Autodesk Inventor part; units mm, degrees
ref_plane "Work Plane1" through (0, -12, 0) normal (0, 1, 0) x (1, 0, 0)
ref_plane "YZ Plane" through (0, 0, 0) normal (1, 0, 0) x (0, 1, 0)
ref_plane "XZ Plane" through (0, 0, 0) normal (0, 1, 0) x (-1, 0, 0)
sketch "Sketch1" plane through (0, 0, 0) normal (0, 1, 0) x (-1, 0, 0)
  line L0 (0, 0) -> (35, 0)
  line L1 (35, 0) -> (35, 40)
  line L2 (35, 40) -> (0, 40)
  line L3 (0, 40) -> (0, 0)
  line L4 (50, 0) -> (85, 0)
  line L5 (85, 0) -> (85, 40)
  line L6 (85, 40) -> (50, 40)
  line L7 (50, 40) -> (50, 0)
  line L8 (50, 40) -> (35, 40)
  line L9 (50, 0) -> (35, 0)
  line L10 (0, 40) -> (0, 51)
  line L11 (0, 51) -> (85, 51)
  line L12 (85, 51) -> (85, 40)
  dimension "d0" = 40
  dimension "d1" = 35
  dimension "d2" = 40
  dimension "d3" = 35
  dimension "d4" = 50
  dimension "d5" = 0
  dimension "d6" = 11
extrude "Extrusion1" add sketch "Sketch1" along normal blind 30
sketch "Sketch2" plane through (0, 0, 0) normal (0, -1, 0) x (1, 0, 0)
  line L0 (-85, 0) -> (-85, 51)
  line L1 (0, 0) -> (-85, 0)
  line L2 (0, 51) -> (0, 0)
  line L3 (-85, 51) -> (0, 51)
  line L4 (-85, 51) -> (0, 51)
  line L5 (-85, 0) -> (-85, 51)
  line L6 (0, 51) -> (-85, 51)
  line L7 (-85, 51) -> (-85, 41)
  line L8 (-85, 41) -> (0, 41)
  line L9 (0, 41) -> (0, 51)
  dimension "d9" = 10
extrude "Extrusion2" add sketch "Sketch2" along normal blind 12 contours L0 L3 L2 L8
sketch "Sketch3" plane through (0, 0, 0) normal (0, 0, -1) x (-1, 0, 0)
  line L0 (0, 0) -> (85, 0)
  line L1 (85, 0) -> (85, 30)
  line L2 (0, 30) -> (85, 30)
  line L3 (0, 0) -> (0, 30)
  circle A0 centre (17.5, 10) radius 5.25
  circle A1 centre (67.5, 10) radius 5.25
  dimension "d12" = 10.5
  dimension "d13" = 10.5
  dimension "d14" = 10
  dimension "d15" = 10
  dimension "d16" = 50
  dimension "d17" = 17.5
  dimension "d18" = 17.5
extrude "Extrusion3" cut sketch "Sketch3" against normal blind 30 contours A0 | A1
sketch "Sketch4" plane through (0, 30, 0) normal (0, 1, 0) x (1, 0, 0)
  line L0 (-85, 0) -> (-85, -51)
  line L1 (-85, -51) -> (0, -51)
  line L2 (0, -51) -> (0, 0)
  line L3 (0, 0) -> (-85, 0)
  line L4 (0, -51) -> (-85, -51)
  line L5 (-42.5, -51) -> (-42.5, 0) construction
  line L6 (0, 0) -> (-85, 0)
  circle A0 centre (11.1, -39.9) radius 3.25
  circle A1 centre (25, -51) radius 6.1 construction
  circle A2 centre (11.1, -39.9) radius 5
  circle A3 centre (11.1, -39.9) radius 11.1
  line L7 (0, -51) -> (11.1, -51)
  line L8 (0, -41) -> (-85, -41)
  line L9 (0, -41) -> (0, 0)
  line L10 (0, 0) -> (20.6053, -34.1677)
  circle A4 centre (-96.1, -39.9) radius 3.25
  circle A5 centre (-110, -51) radius 6.1 construction
  circle A6 centre (-96.1, -39.9) radius 5
  circle A7 centre (-96.1, -39.9) radius 11.1
  line L11 (-85, -51) -> (-96.1, -51)
  line L12 (-85, 0) -> (-105.6053, -34.1677)
  dimension "d22" = 6.5
  dimension "d23" = 11.1
  dimension "d24" = 12.2
  dimension "d25" = 25
  dimension "d26" = 0
  dimension "d27" = 10
  dimension "d28" = 11.1
  dimension "d30" = 22.2
extrude "Extrusion4" add sketch "Sketch4" against normal blind 10 contours L0 A7 L12 | A7 | L0 L11 A7 | L10 A3 L2 | A3 L7 L2 | A3 | A2 | A6
ref_plane "Work Plane1" through (0, -12, 0) normal (0, 1, 0) x (1, 0, 0)
sketch "Sketch5" plane through (0, -12, 0) normal (0, 1, 0) x (1, 0, 0)
  arc A0 (11.1, -51) -> (20.6053, -34.1677) centre (11.1, -39.9) ccw
  circle A1 centre (11.1, -39.9) radius 3.25
  line L0 (0, -41) -> (0, -51)
  line L1 (0, -41) -> (0, 0)
  circle A2 centre (11.1, -39.9) radius 3.25
  circle A3 centre (11.1, -39.9) radius 11.1
  line L2 (11.1, -51) -> (0, -51)
  line L3 (-85, -41) -> (0, -41)
  arc A4 (-105.6053, -34.1677) -> (-96.1, -51) centre (-96.1, -39.9) ccw
  circle A5 centre (-96.1, -39.9) radius 3.25
  line L4 (-85, -51) -> (-96.1, -51)
  line L5 (-85, -51) -> (-85, -41)
  line L6 (-85, 0) -> (-85, -41)
  circle A6 centre (-96.1, -39.9) radius 11.1
  point P0 (20.6053, -34.1677)
  point P1 (0, -39.9)
  point P2 (-85, -39.9)
  point P3 (-105.6053, -34.1677)
extrude "Extrusion5" add sketch "Sketch5" along normal blind 10
sketch "Sketch6" plane through (0, 30, 0) normal (0, 1, 0) x (1, 0, 0)
  circle A0 centre (-96.1, -39.9) radius 3.25
  circle A1 centre (11.1, -39.9) radius 3.25
  circle A2 centre (11.1, -39.9) radius 5.75
  circle A3 centre (-96.1, -39.9) radius 5.75
  point P0 (0, 0)
  dimension "d36" = 11.5
  dimension "d37" = 11.5
extrude "Extrusion6" cut sketch "Sketch6" against normal blind 4
sketch "Sketch7" plane through (0, -12, 0) normal (0, -1, 0) x (1, 0, 0)
  circle A0 centre (11.1, 39.9) radius 3.25
  circle A1 centre (-96.1, 39.9) radius 3.25
  circle A2 centre (11.1, 39.9) radius 5.75
  circle A3 centre (11.1, 39.9) radius 5.75
  circle A4 centre (-96.1, 39.9) radius 5.75
  point P0 (0, 0)
extrude "Extrusion7" cut sketch "Sketch7" against normal blind 4
sketch "Sketch8" plane through (0, 0, 0) normal (0, -1, 0) x (1, 0, 0)
  line L0 (0, 41) -> (-85, 41)
  line L1 (-85, 0) -> (-85, 41)
  line L2 (0, 0) -> (-85, 0)
  line L3 (0, 41) -> (0, 0)
  circle A0 centre (-7.5, 6) radius 2.25
  circle A1 centre (-27.5, 6) radius 2.25
  circle A2 centre (-7.5, 34) radius 2.25
  circle A3 centre (-27.5, 34) radius 2.25
  line L4 (0, 0) -> (-85, 0)
  line L5 (-42.5, 0) -> (-42.5, 41) construction
  line L6 (-85, 41) -> (0, 41)
  circle A4 centre (-77.5, 6) radius 2.25
  circle A5 centre (-57.5, 6) radius 2.25
  circle A6 centre (-77.5, 34) radius 2.25
  circle A7 centre (-57.5, 34) radius 2.25
  dimension "d42" = 4.5
  dimension "d45" = 20
  dimension "d48" = 28
  dimension "d51" = 6
  dimension "d52" = 7.5
extrude "Extrusion8" cut sketch "Sketch8" against normal through all contours A0 | A1 | A2 | A3 | A4 | A5 | A6 | A7
sketch "Sketch9" plane through (0, 30, 0) normal (0, 1, 0) x (1, 0, 0)
  line L0 (-12.25, 0) -> (-12.25, -30)
  circle A0 centre (-7.5, -34) radius 2.25
  circle A1 centre (-77.5, -6) radius 2.25
  circle A2 centre (-57.5, -6) radius 2.25
  circle A3 centre (-7.5, -6) radius 2.25
  circle A4 centre (-27.5, -34) radius 2.25
  circle A5 centre (-77.5, -34) radius 2.25
  circle A6 centre (-57.5, -34) radius 2.25
  circle A7 centre (-27.5, -6) radius 2.25
  circle A8 centre (-96.1, -39.9) radius 5.75
  circle A9 centre (11.1, -39.9) radius 5.75
  line L1 (-96.1, -51) -> (11.1, -51)
  arc A10 (11.1, -51) -> (20.6053, -34.1677) centre (11.1, -39.9) ccw
  line L2 (20.6053, -34.1677) -> (0, 0)
  line L3 (0, 0) -> (-85, 0)
  line L4 (-85, 0) -> (-105.6053, -34.1677)
  arc A11 (-105.6053, -34.1677) -> (-96.1, -51) centre (-96.1, -39.9) ccw
  circle A12 centre (-7.5, -6) radius 4.5
  circle A13 centre (-7.5, -34) radius 4.5
  circle A14 centre (-27.5, -34) radius 2.25
  circle A15 centre (-27.5, -34) radius 4.5
  circle A16 centre (-27.5, -6) radius 2.25
  circle A17 centre (-27.5, -6) radius 4.5
  circle A18 centre (-57.5, -6) radius 2.25
  circle A19 centre (-57.5, -6) radius 4.5
  circle A20 centre (-57.5, -34) radius 4.5
  circle A21 centre (-77.5, -34) radius 2.25
  circle A22 centre (-77.5, -34) radius 4.5
  circle A23 centre (-77.5, -6) radius 2.25
  circle A24 centre (-77.5, -6) radius 4.5
  dimension "d55" = 9
  dimension "d56" = 9
  dimension "d57" = 9
  dimension "d58" = 9
  dimension "d59" = 9
  dimension "d60" = 9
  dimension "d61" = 9
  dimension "d62" = 9
extrude "Extrusion9" cut sketch "Sketch9" against normal blind 20 contours A0 | A1 | A2 | A3 | A4 | A5 | A6 | A7 | A12 | A13 | A15 | A17 | A19 | A20 | A22 | A24
equation "\"d17\" = d18"
equation "\"d23\" = 0.5 * d30"
equation "\"d28\" = 0.5 * d27 + 0.5 * d24"
equation "\"d30\" = 2 * d28"
equation "\"d31\" = d27"
equation "\"d56\" = d55"
equation "\"d57\" = d55"
equation "\"d58\" = d55"
equation "\"d59\" = d55"
equation "\"d60\" = d55"
equation "\"d61\" = d55"
equation "\"d62\" = d55"
properties part number "YAxisEndBlock_10mm"
Geometry: final body of the model. Coordinates: model frame, mm. A direction names the side the tool comes from. Round coordinates to 2 decimals unless told otherwise and drop trailing zeros. Loops run counter-clockwise (first coordinate to the right, second up) from the corner with the lowest first, then second, coordinate; pieces in that order, holes last. Notation, with made-up numbers: (57.25, 61.25) -> (99.25, 61.25) arc R12 cw to (99.25, 76.25) -> close; hole circle Ø3 at (73, 81). An arc over 180 degrees is marked (long way). Write each question's results on one line, items separated by ' | '.
Item 1: Set-up query: faces 4 (the face through (-42, 0, 21)), 5 (the face through (18.69, -7.07, 31.8)), 6 (the face through (14, 26, 42)). Return all of +Z, -Z, +X, -X, +Y, -Y with unobstructed straight access to the full face (end or side cutting, diameter ignored); none if empty.
Answers below:
face 4: -Z, +X, -X, -Y | face 5: -Y | face 6: +Y
Item 2: Cut plane B-B on y = 2. State how many separate pieces and enclosed holes the cut face has, and give its area (3 significant figures).
Answers below:
separate pieces: 1 | enclosed holes: 8 | area: 4,210 mm²
Item 3: Pull-direction query (Y, two-part tool) for faces 1 (the face through (-80, 10, 35)), 2 (the face through (-99.347, 23.042, 39.757)), 3 (the face through (-85, 9, 25)); classes: pulls with the +Y half, pulls with the -Y half, needs draft (parallel to the pull), parting line crosses it, or undercut.
Answers below:
face 1: pulls with the +Y half | face 2: needs draft | face 3: undercut
Item 4: Line query: probe 1 along X at (y, z) = (-4.4, 39.9); probe 2 along Z at (x, y) = (-7, 20); probe 3 along Z at (x, y) = (-57.5, 6.25). Output: solid intervals per line, ascending. Write a range as [from, to].
Answers below:
probe 1: x = [-107.2, -99.35], [-92.85, -85], [0, 7.85], [14.35, 22.2] | probe 2: z = [0, 1.53], [10.47, 29.53], [38.47, 51] | probe 3: z = [0, 3.75], [8.25, 31.75], [36.25, 51]
Item 5: Cut plane A-A on x = -77.5. Return the cut outline in (y, z).
Answers below:
outline: (-12, 41) -> (0, 41) -> (0, 36.25) -> (10, 36.25) -> (10, 38.5) -> (30, 38.5) -> (30, 51) -> (-12, 51) -> close; (0, 0) -> (30, 0) -> (30, 1.5) -> (10, 1.5) -> (10, 3.75) -> (0, 3.75) -> close; (0, 8.25) -> (10, 8.25) -> (10, 10.5) -> (30, 10.5) -> (30, 29.5) -> (10, 29.5) -> (10, 31.75) -> (0, 31.75) -> close
Item 6: Pin query (flat end, axial travel): pin 1 Ø7 at (x, z) = (-96.1, 39.9) entering from +Y; pin 2 Ø1.5 at (x, z) = (-91, 16) entering from -Y; pin 3 Ø7 at (x, z) = (-27.5, 6) entering from +Y. Return the tip coordinate at first contact, or that it passes through.
Answers below:
pin 1: stops at y = 26 | pin 2: stops at y = 20 | pin 3: stops at y = 10
Item 7: Cut plane C-C on z = 24. Return the cut outline in (x, y), and give its area (3 significant figures).
Answers below:
outline: (-99.47, 20) -> (-85, 20) -> (-85, 0) -> (0, 0) -> (0, 20) -> (14.47, 20) -> (14.47, 30) -> (-99.47, 30) -> close; hole circle Ø10.5 at (-67.5, 10); hole circle Ø10.5 at (-17.5, 10) | area: 2,670 mm²
